Check sheet for the modelled part. Datum: model origin and axes. Units: mm. A direction names the side the tool comes from. Coordinates: 2 decimals unless noted, no trailing zeros. Loops run counter-clockwise (first coordinate to the right, second up) from the corner with the lowest first, then second, coordinate; pieces in that order, holes last. Notation, with made-up numbers: (-40, 6) - (-28, 6) arc R22 ccw to (-28, 28) - close; hole circle Ø11 at (38.25, -30.75). An arc over 180 degrees is marked (long way). Answer as a JSON object with one key per item and string values. Group by question number.
from build123d import *

# Parameters (mm, degrees)
SKETCH_1_R          = 2.3
EXTRUDE_1_DEPTH     = 1
SKETCH_2_R          = 2
EXTRUDE_2_DEPTH     = 5
SKETCH_3_W          = 0.5
SKETCH_3_H          = 0.5
EXTRUDE_3_DEPTH     = 3
SKETCH_4_W          = 9.434244616
SKETCH_4_H          = 19.451997256
CUT_EXTRUDE_1_DEPTH = 3
FILLET_1_R          = 2


with BuildPart() as part:
    # Эскиз1 → Бобышка-Вытянуть1 (new body)
    with BuildSketch(Plane(origin=(0, 0, 0), x_dir=(1, 0, 0), z_dir=(0, 1, 0))):
        with Locations(Location((0, 0, 0), (0, 0, 270))):
            Circle(SKETCH_1_R)
    extrude(amount=EXTRUDE_1_DEPTH)

    # Эскиз2 → Бобышка-Вытянуть2 (add)
    with BuildSketch(Plane(origin=(0, 1, 0), x_dir=(1, 0, 0), z_dir=(0, 1, 0))):
        with Locations(Location((0, 0, 0), (0, 0, 270))):
            Circle(SKETCH_2_R)
    extrude(amount=EXTRUDE_2_DEPTH)

    # Эскиз3 → Бобышка-Вытянуть3 (add)
    with BuildSketch(Plane.XZ):
        with Locations((0, 1.27)):
            Rectangle(SKETCH_3_W, SKETCH_3_H)
    extrude_3 = extrude(amount=EXTRUDE_3_DEPTH)

    # Зеркальное отражение1: Бобышка-Вытянуть3 across plane
    add(extrude_3.mirror(Plane(origin=(0, 0, 0), x_dir=(1, 0, 0), z_dir=(0, 0, -1))))

    # Эскиз4 → Вырез-Вытянуть1 (cut)
    with BuildSketch(Plane.XY.offset(2)):
        Rectangle(SKETCH_4_W, SKETCH_4_H)
    extrude(amount=CUT_EXTRUDE_1_DEPTH, mode=Mode.SUBTRACT)

    # Скругление1
    fillet_1_edges = [part.edges().sort_by_distance(p)[0] for p in [
        (0, 6, -2),
    ]]
    fillet(fillet_1_edges, radius=FILLET_1_R)


solid = part.part
1. Sectioned sample at A-A on y = -1.25. Record the cut outline in (x, z).
2. Sectioned sample at D-D on y = 1.25. Record the cut outline in (x, z).
3. Material ranges on line 1 (Z direction, x = 0.1, y = 2); line 2 (Y direction, x = 1.7, z = 1.5), recorded low to high.
4. Sectioned sample at B-B on z = 0. Record the cut outline in (x, y).
5. Gauge pin test, flat ends, axial feed: pin 1 (2 mm diameter, centred on y = -0.5, z = 0.5, fed in from +X); pin 2 (1 mm diameter, centred on y = 3, z = 0.5, fed in from +X); pin 3 (0.6 mm diameter, centred on y = -2, z = -1.5, fed in from +X); pin 4 (1.5 mm diameter, centred on x = 1, y = 4.5, fed in from +Z). Record the tip position at first contact, or that the pin passes through.
6. Access from +Z, -Z, +X, -X, +Y, -Y to the whole of each face (thin tool, end or side, straight path). Record for faces 1 (the face through (0.08, 0.49, -2.3)), 2 (the face through (-2, 2, 0)).
7. Sectioned sample at C-C on x = 1.6. Record the cut outline in (y, z).
Answers follow:
{
 "1": {"outline": "(-0.25, -1.52) - (0.25, -1.52) - (0.25, -1.02) - (-0.25, -1.02) - close; (-0.25, 1.02) - (0.25, 1.02) - (0.25, 1.52) - (-0.25, 1.52) - close"},
 "2": {"outline": "circle Ø4 at (0, 0)"},
 "3": {"line 1": "z = -2 to 2", "line 2": "y = 0 to 1"},
 "4": {"outline": "(-2.3, 0) - (2.3, 0) - (2.3, 1) - (2, 1) - (2, 4) arc R2 ccw to (-2, 4) - (-2, 1) - (-2.3, 1) - close"},
 "5": {"pin 1": "stops at x = 2.3", "pin 2": "stops at x = 2", "pin 3": "stops at x = 0.25", "pin 4": "stops at z = 1.97"},
 "6": {"face 1": "+Y, -Y", "face 2": "+Y"},
 "7": {"outline": "(0, -1.65) - (1, -1.65) - (1, -1.2) - (4, -1.2) arc R1.2 ccw to (4, 1.2) - (1, 1.2) - (1, 1.65) - (0, 1.65) - close"}
}
